```python
from build123d import *

# Parameters (mm, degrees)
F1_DEPTH  = 40
F2_R      = 10
F2_R_2    = 5
F1_FACE_W = 40
F1_FACE_H = 35
F3_DEPTH  = 18


with BuildPart() as f1:
    # F0 (on Right) → F1 (new body)
    with BuildSketch(Plane.YZ):
        Polygon((12.356097, 23.456169), (12.356097, 11.191107), (-12.643903, 11.191107), (-12.643903, -23.808893), (12.356097, -23.808893), (12.356097, -36.119621), (17.700054, -36.119621), (17.700054, 23.456169), align=None)
    extrude(amount=F1_DEPTH)

    # F2 (on Front) + F1_face (on face) → F3 (join)
    with BuildSketch(Plane.XZ):
        with Locations((19.120954, -4.390738)):
            Circle(F2_R)
        with Locations((19.120954, -4.390738)):
            Circle(F2_R_2, mode=Mode.SUBTRACT)
    with BuildSketch(Plane(origin=(20, -12.643903, -6.308893), x_dir=(1, 0, 0), z_dir=(0, -1, 0))):
        Rectangle(F1_FACE_W, F1_FACE_H)
    extrude(amount=-F3_DEPTH)


solid = f1.part
```
The model under review builds one solid part; all positions refer to its coordinate system, in mm. A direction names the side the tool comes from. Round coordinates to 2 decimals unless told otherwise and drop trailing zeros. Write each loop counter-clockwise with the first axis right and the second up, starting at its lowest first coordinate (ties: lowest second). Pieces come first, ordered by that corner, then holes. Notation, with made-up numbers: (20.25, 10.5) - (74.25, 10.5) arc R13 ccw to (74.25, 23.5) - close; hole circle Ø8 at (-36, -24). An arc over 180 degrees is marked (long way). One line per question, with ' | ' between items.
Item 1: Add section A-A, the plane x = 37.5. Give the boundary of the cut face in (y, z), then the cut area to 3 significant figures.
Resolved:
outline: (-12.64, -23.81) - (12.36, -23.81) - (12.36, -36.12) - (17.7, -36.12) - (17.7, 23.46) - (12.36, 23.46) - (12.36, 11.19) - (-12.64, 11.19) - close | area: 1,190 mm2
Item 2: Add section B-B, the plane y = 2.5. Give the boundary of the cut face in (x, z).
Resolved:
outline: (0, -23.81) - (40, -23.81) - (40, 11.19) - (0, 11.19) - close
Item 3: Add section D-D, the plane x = 20. Give the boundary of the cut face in (y, z).
Resolved:
outline: (-12.64, -23.81) - (12.36, -23.81) - (12.36, -36.12) - (17.7, -36.12) - (17.7, -14.35) - (18, -14.35) - (18, -9.31) - (17.7, -9.31) - (17.7, 0.53) - (18, 0.53) - (18, 5.57) - (17.7, 5.57) - (17.7, 23.46) - (12.36, 23.46) - (12.36, 11.19) - (-12.64, 11.19) - close
Item 4: For faces 1 (the face through (20, 12.356, 17)), 2 (the face through (40, 6, -6)), 3 (the face through (20, 12.356, -30)), list the 3-axis set-ups (+Z, -Z, +X, -X, +Y, -Y) from which the entire face can be reached by the end or side of a thin tool; tool diameter is ignored.
Resolved:
face 1: +Z, +X, -X, -Y | face 2: +Z, -Z, +X, +Y, -Y | face 3: -Z, +X, -X, -Y
Item 5: Add section C-C, the plane z = -28.5. Give the boundary of the cut face in (x, y).
Resolved:
outline: (0, 12.36) - (40, 12.36) - (40, 17.7) - (0, 17.7) - close
Item 6: For P1, Ø2, axis at x = 32.5, z = -26.5, coming from the +Y side; P2, Ø1.5, axis at x = 17.5, y = 10.5, coming from the -Z side; P3, Ø12.5, axis at x = 24, y = -2, coming from the +Z side, all flat-tipped, find the tip position at first contact; note any pin that passes through.
Resolved:
P1: stops at y = 17.7 | P2: stops at z = -23.81 | P3: stops at z = 11.19
Item 7: To check wall thickness, follow probe 1 along Y at (x, z) = (29.5, -21); probe 2 along Z at (x, y) = (26, -11); probe 3 along Y at (x, z) = (14, -28). State the ranges of each line that lie inside material, in increasing order.
Resolved:
probe 1: y = -12.64 to 17.7 | probe 2: z = -23.81 to 11.19 | probe 3: y = 12.36 to 17.7
Item 8: The part is to be moulded in two halves that separate along X. For faces 4 (the face through (24.2, 17.7, -13.4)), 5 (the face through (19, 17.7, -4)), 6 (the face through (0, 6, -6)), say which applies: pulls with the +X half, pulls with the -X half, needs draft (parallel to the pull), parting line crosses it, or undercut.
Resolved:
face 4: needs draft | face 5: undercut | face 6: pulls with the -X half
